Answer from the drawing. Dimensions are ordinates in mm from the lowest x, y and z of the part. A direction names the side the tool comes from. Give positions to 0.01 mm unless a question says otherwise; leave off trailing zeros. Order: outer loops, then holes, each group sorted by start corner. A loop starts at its lowest first (then second) coordinate and runs counter-clockwise, first axis right, second up.
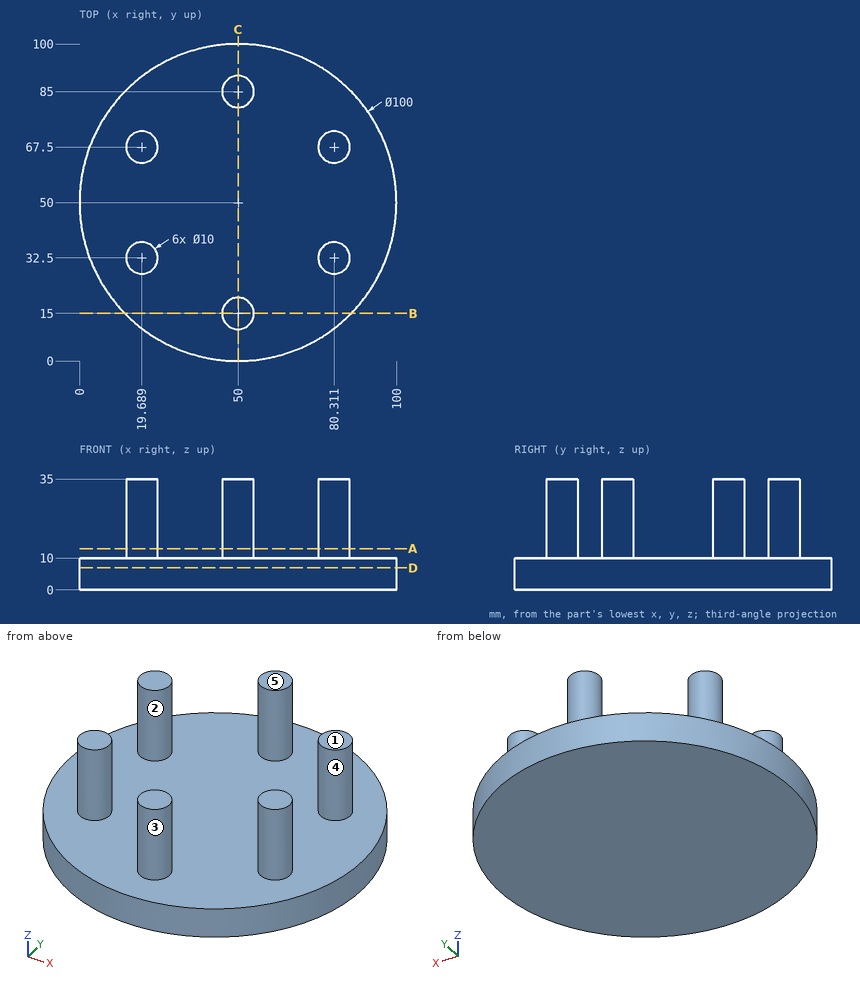
1. The part is cut by section D-D (z = 7). Write down the section's boundary in (x, y), then the cut area to 3 significant figures.
Findings below:
outline: circle Ø100 at (50, 50)
area: 7,850 mm2
2. The part is cut by section B-B (y = 15). Write down the section's boundary in (x, z), then the cut area to 3 significant figures.
Findings below:
outline: (14.29, 0) - (85.71, 0) - (85.71, 10) - (55, 10) - (55, 35) - (45, 35) - (45, 10) - (14.29, 10) - close
area: 964 mm2
3. The mould has two halves that part along X. Classify the marked faces 3, 4 and 5: pulls with the +X half, pulls with the -X half, needs draft (parallel to the pull), parting line crosses it, or undercut.
Findings below:
face 3: parting line crosses it
face 4: undercut
face 5: needs draft
4. Which of the six approach directions +Z, -Z, +X, -X, +Y, -Y give full straight-line access (tool end or side, diameter ignored) to the marked faces 1 and 2?
Findings below:
face 1: +Z, +X, -X, +Y, -Y
face 2: +Z
5. Straight lines are drawn through the part: probe 1 along Z at (x, y) = (44.5, 48.5); probe 2 along X at (y, z) = (65.5, 19); probe 3 along Y at (x, z) = (81.5, 28). For each, find the intervals that lie inside material, in ascending order.
Findings below:
probe 1: z = 0 to 10
probe 2: x = 15.11 to 24.27, 75.73 to 84.89
probe 3: y = 27.64 to 37.36, 62.64 to 72.36
6. The part is cut by section A-A (z = 13). Write down the section's boundary in (x, y), then the cut area to 3 significant figures.
Findings below:
outline: circle Ø10 at (19.69, 32.5); circle Ø10 at (19.69, 67.5); circle Ø10 at (50, 15); circle Ø10 at (50, 85); circle Ø10 at (80.31, 32.5); circle Ø10 at (80.31, 67.5)
area: 471 mm2
7. The part is cut by section C-C (x = 50). Write down the section's boundary in (y, z), then the cut area to 3 significant figures.
Findings below:
outline: (0, 0) - (100, 0) - (100, 10) - (90, 10) - (90, 35) - (80, 35) - (80, 10) - (20, 10) - (20, 35) - (10, 35) - (10, 10) - (0, 10) - close
area: 1,500 mm2
8. Given P1, Ø3, axis at y = 90, z = 30.5, coming from the +X side; P2, Ø1.5, axis at x = 62.5, z = 4, coming from the +Y side; P3, Ø1, axis at y = 36.5, z = 11.5, coming from the -X side; P4, Ø8, axis at x = 69.5, z = 16.5, coming from the -Y side, each flat-ended and moving along its own axis, determine where each tip first touches the part or whether it passes through.
Findings below:
P1: stops at x = 53.57
P2: stops at y = 98.6
P3: stops at x = 16.12
P4: passes through
